Here's how the part is built. I have some questions about the finished solid (model axes, mm). A direction names the side the tool comes from. Coordinates: 2 decimals unless noted, no trailing zeros. Loops run counter-clockwise (first coordinate to the right, second up) from the corner with the lowest first, then second, coordinate; pieces in that order, holes last. Notation, with made-up numbers: (39, 34) - (67, 34) arc R34 cw to (67, 70) - close; hole circle Ø1 at (25, 55). An arc over 180 degrees is marked (long way). Use a Markdown table: item, result.
```python
from build123d import *

# Parameters (mm, degrees)
F0_W     = 101.6
F0_H     = 127
F0_R     = 9.525
F0_W_2   = 50.8
F0_H_2   = 50.8
F0_R_2   = 6.35
F1_DEPTH = 19.05
F2_R     = 12.7
F3_R     = 6.35
F4_DEPTH = 101.601


with BuildPart() as f1:
    # F0 (on Top) → F1 (new body)
    with BuildSketch(Plane.XY):
        with Locations((-89.981672, 0)):
            Rectangle(F0_W, F0_H)
        with Locations((-121.731672, -44.45)):
            Circle(F0_R, mode=Mode.SUBTRACT)
        with Locations((-58.231672, -44.45)):
            Circle(F0_R, mode=Mode.SUBTRACT)
        with Locations((-121.731672, 44.45)):
            Circle(F0_R, mode=Mode.SUBTRACT)
        with Locations((-89.981672, 0)):
            Rectangle(F0_W_2, F0_H_2, mode=Mode.SUBTRACT)
        with Locations((-58.231672, 44.45)):
            Circle(F0_R_2, mode=Mode.SUBTRACT)
    extrude(amount=F1_DEPTH)

    # F2
    f2_edges = [f1.edges().sort_by_distance(p)[0] for p in [
        (-115.381672, -25.4, 9.525),
        (-64.581672, -25.4, 9.525),
        (-64.581672, 25.4, 9.525),
        (-115.381672, 25.4, 9.525),
    ]]
    fillet(f2_edges, radius=F2_R)

    # F3 (on face) → F4 (cut, through all)
    with BuildSketch(Plane.YZ.offset(-39.181672)):
        with Locations((0, 9.525)):
            Circle(F3_R)
    extrude(amount=-F4_DEPTH, mode=Mode.SUBTRACT)


solid = f1.part
```
Q1. Will this pin go through, and if not, where does the flat tip stop? P1, Ø10, axis at x = -58.23, y = 44.45, coming from the -Z side.
Check values:
| item | result |
|---|---|
| P1 | through |
Q2. Please list where these lines run through material, in increasing order: L1, parallel to Y at x = -96.5, z = 4; L2, parallel to Y at x = -121, z = 9.75; L3, parallel to X at y = 9, z = 14.25. Write a range as from..to.
Check values:
| item | result |
|---|---|
| L1 | -63.5..-25.4, 25.4..63.5 |
| L2 | -63.5..-53.95, -34.95..-6.35, 6.35..34.95, 53.95..63.5 |
| L3 | -140.78..-115.38, -64.58..-39.18 |
Q3. I want a section at B-B, the plane z = 5.5. Write out the boundary of the cut face in (x, y) (3 decimals), then the cut area to 3 significant figures.
Check values:
| item | result |
|---|---|
| outline | (-140.782, -63.5) - (-39.182, -63.5) - (-39.182, -4.911) - (-64.582, -4.911) - (-64.582, -12.7) arc R12.7 cw to (-77.282, -25.4) - (-102.682, -25.4) arc R12.7 cw to (-115.382, -12.7) - (-115.382, -4.911) - (-140.782, -4.911) - close; (-140.782, 4.911) - (-115.382, 4.911) - (-115.382, 12.7) arc R12.7 cw to (-102.682, 25.4) - (-77.282, 25.4) arc R12.7 cw to (-64.582, 12.7) - (-64.582, 4.911) - (-39.182, 4.911) - (-39.182, 63.5) - (-140.782, 63.5) - close; hole circle Ø19.05 at (-121.732, -44.45); hole circle Ø19.05 at (-121.732, 44.45); hole circle Ø19.05 at (-58.232, -44.45); hole circle Ø12.7 at (-58.232, 44.45) |
| area | 8,980 mm^2 |
Q4. I want a section at D-D, the plane y = 44.45. Write out the boundary of the cut face in (x, z).
Check values:
| item | result |
|---|---|
| outline | (-140.78, 0) - (-131.26, 0) - (-131.26, 19.05) - (-140.78, 19.05) - close; (-112.21, 0) - (-64.58, 0) - (-64.58, 19.05) - (-112.21, 19.05) - close; (-51.88, 0) - (-39.18, 0) - (-39.18, 19.05) - (-51.88, 19.05) - close |
Q5. Which directions (+Z, -Z, +X, -X, +Y, -Y) give clear straight access to the entire face, cutting with the end or side of a thin tool? Please do faces 1 (the face through (-68.2, 21.58, 9.66)), 2 (the face through (-39.182, -1, 3)).
Check values:
| item | result |
|---|---|
| face 1 | +Z, -Z |
| face 2 | +Z, -Z, +X, +Y, -Y |
Q6. If we mould it in two halves opening along Z, with no side actions, what happens to faces 3 (the face through (-51.704, -1.377, 3.326)), 4 (the face through (-115.382, 0, 3)), 5 (the face through (-91, 29, 19.05)), 6 (the face through (-91, 29, 0))? For each: pulls with the +Z half, pulls with the -Z half, needs draft (parallel to the pull), parting line crosses it, or undercut.
Check values:
| item | result |
|---|---|
| face 3 | undercut |
| face 4 | needs draft |
| face 5 | pulls with the +Z half |
| face 6 | pulls with the -Z half |
Q7. I want a section at C-C, the plane x = -95. Write out the boundary of the cut face in (y, z), then the cut area to 3 significant figures.
Check values:
| item | result |
|---|---|
| outline | (-63.5, 0) - (-25.4, 0) - (-25.4, 19.05) - (-63.5, 19.05) - close; (25.4, 0) - (63.5, 0) - (63.5, 19.05) - (25.4, 19.05) - close |
| area | 1,450 mm^2 |
Q8. I want a section at A-A, the plane y = 0. Write out the boundary of the cut face in (x, z) (3 decimals).
Check values:
| item | result |
|---|---|
| outline | (-140.782, 0) - (-115.382, 0) - (-115.382, 3.175) - (-140.782, 3.175) - close; (-140.782, 15.875) - (-115.382, 15.875) - (-115.382, 19.05) - (-140.782, 19.05) - close; (-64.582, 0) - (-39.182, 0) - (-39.182, 3.175) - (-64.582, 3.175) - close; (-64.582, 15.875) - (-39.182, 15.875) - (-39.182, 19.05) - (-64.582, 19.05) - close |
